Here's how the part is built. I have some questions about the finished solid (model axes, mm). A direction names the side the tool comes from. Coordinates: 2 decimals unless noted, no trailing zeros. Loops run counter-clockwise (first coordinate to the right, second up) from the corner with the lowest first, then second, coordinate; pieces in that order, holes last. Notation, with made-up numbers: M 57,-38 L 105,-38 A16 ccw 105,-11 Z; hole C 56.5,60 d3. An arc over 180 degrees is marked long. Use one line per item in the form item = value. Start each with the question number.
(1) Will this pin go through, and if not, where does the flat tip stop? P1, Ø3.5, axis at x = 41.25, y = -100.5, coming from the +Z side.
(2) Imagine slicing it at A-A, the plane x = 5. Please give me the cut outline in (y, z).
(3) Imagine slicing it at D-D, the plane y = 14.5. Please give me the cut outline in (x, z), and give its area (3 significant figures).
(4) Please list where these lines run through material, in increasing order: L1, parallel to Y at x = 11, z = 1.7; L2, parallel to X at y = -132, z = 0.8; L3, parallel to X at y = 100, z = 0.6.
(5) Imagine slicing it at C-C, the plane z = 2.55. State how many separate pieces and enclosed holes the cut face has, and give its area (3 significant figures).
(6) On a 3-axis mill with a long thin cutter (end or side, diameter ignored), from which of +Z, -Z, +X, -X, +Y, -Y can I reach the whole of each face in a straight line? I mean faces 1 (the flat face through (-37, 3, 0)), 2 (the cylindrical face through (37.591, 9.888, 1.479)). Say none if no direction works.
(7) Thinking about a two-plate mould opening in Y: for faces 3 (the flat face through (-37, 3, 3)), 4 (the cylindrical face through (-37.362, 9.659, 1.479)), which applies, +Y half, -Y half, draft (parallel to the pull), parting line (faces both ways), or undercut?
(8) Imagine slicing it at B-B, the plane y = -57. Please give me the cut outline in (x, z).
Autodesk Inventor part; units mm, degrees
ref_plane "YZ Plane" through (0, 0, 0) normal (1, 0, 0) x (0, 1, 0)
ref_plane "XZ Plane" through (0, 0, 0) normal (0, 1, 0) x (-1, 0, 0)
ref_plane "XY Plane" through (0, 0, 0) normal (0, 0, 1) x (1, 0, 0)
sketch "スケッチ1" plane through (0, 0, 0) normal (0, 0, 1) x (1, 0, 0)
  line L0 (-55, -215) -> (55, -215)
  line L1 (55, -215) -> (55, 215)
  line L2 (55, 215) -> (-55, 215)
  line L3 (-55, 215) -> (-55, -215)
  line L4 (-55, -215) -> (55, 215) construction
  line L5 (55, -215) -> (-55, 215) construction
  line L6 (-55, 185) -> (-50, 185) construction
  line L7 (-50, 185) -> (-25, 210) construction
  line L8 (-25, 210) -> (-25, 215) construction
  line L9 (-46, 95.75) -> (46, 95.75) construction
  line L10 (46, 95.75) -> (46, 187.75) construction
  line L11 (46, 187.75) -> (-46, 187.75) construction
  line L12 (-46, 187.75) -> (-46, 95.75) construction
  line L13 (-46, 95.75) -> (46, 187.75) construction
  line L14 (46, 95.75) -> (-46, 187.75) construction
  line L15 (-46, 1.25) -> (46, 1.25) construction
  line L16 (46, 1.25) -> (46, 93.25) construction
  line L17 (46, 93.25) -> (-46, 93.25) construction
  line L18 (-46, 93.25) -> (-46, 1.25) construction
  line L19 (-46, 1.25) -> (46, 93.25) construction
  line L20 (46, 1.25) -> (-46, 93.25) construction
  line L21 (0, 0) -> (0, 141.75) construction
  circle A0 centre (0, 141.75) radius 53 construction
  line L22 (-44.7, 97.05) -> (44.7, 97.05) construction
  line L23 (44.7, 97.05) -> (44.7, 186.45) construction
  line L24 (44.7, 186.45) -> (-44.7, 186.45) construction
  line L25 (-44.7, 186.45) -> (-44.7, 97.05) construction
  line L26 (-44.7, 97.05) -> (44.7, 186.45) construction
  line L27 (44.7, 97.05) -> (-44.7, 186.45) construction
  arc A1 (-28.4765, 186.45) -> (-44.7, 170.2265) centre (0, 141.75) ccw
  arc A2 (-44.7, 113.2735) -> (-28.4765, 97.05) centre (0, 141.75) ccw
  arc A3 (28.4765, 97.05) -> (44.7, 113.2735) centre (0, 141.75) ccw
  arc A4 (44.7, 170.2265) -> (28.4765, 186.45) centre (0, 141.75) ccw
  line L28 (-28.4765, 186.45) -> (28.4765, 186.45)
  line L29 (-44.7, 170.2265) -> (-44.7, 113.2735)
  line L30 (-28.4765, 97.05) -> (28.4765, 97.05)
  line L31 (44.7, 113.2735) -> (44.7, 170.2265)
  line L32 (-41.25, 100.5) -> (41.25, 100.5) construction
  line L33 (41.25, 100.5) -> (41.25, 183) construction
  line L34 (41.25, 183) -> (-41.25, 183) construction
  line L35 (-41.25, 183) -> (-41.25, 100.5) construction
  line L36 (-41.25, 100.5) -> (41.25, 183) construction
  line L37 (41.25, 100.5) -> (-41.25, 183) construction
  circle A5 centre (-41.25, 183) radius 2.25
  circle A6 centre (-41.25, 100.5) radius 2.25
  circle A7 centre (41.25, 100.5) radius 2.25
  circle A8 centre (41.25, 183) radius 2.25
  circle A9 centre (-41.25, 88.5) radius 2.25
  arc A10 (-28.4765, 91.95) -> (-44.7, 75.7265) centre (0, 47.25) ccw
  line L38 (-28.4765, 91.95) -> (28.4765, 91.95)
  arc A11 (44.7, 75.7265) -> (28.4765, 91.95) centre (0, 47.25) ccw
  circle A12 centre (41.25, 88.5) radius 2.25
  line L39 (44.7, 18.7735) -> (44.7, 75.7265)
  arc A13 (28.4765, 2.55) -> (44.7, 18.7735) centre (0, 47.25) ccw
  circle A14 centre (41.25, 6) radius 2.25
  line L40 (-28.4765, 2.55) -> (28.4765, 2.55)
  circle A15 centre (-41.25, 6) radius 2.25
  arc A16 (-44.7, 18.7735) -> (-28.4765, 2.55) centre (0, 47.25) ccw
  line L41 (-44.7, 75.7265) -> (-44.7, 18.7735)
  circle A17 centre (-41.25, -6) radius 2.25
  arc A18 (-28.4765, -2.55) -> (-44.7, -18.7735) centre (0, -47.25) ccw
  line L42 (-28.4765, -2.55) -> (28.4765, -2.55)
  arc A19 (44.7, -18.7735) -> (28.4765, -2.55) centre (0, -47.25) ccw
  circle A20 centre (41.25, -6) radius 2.25
  line L43 (44.7, -75.7265) -> (44.7, -18.7735)
  arc A21 (28.4765, -91.95) -> (44.7, -75.7265) centre (0, -47.25) ccw
  circle A22 centre (41.25, -88.5) radius 2.25
  line L44 (-28.4765, -91.95) -> (28.4765, -91.95)
  circle A23 centre (-41.25, -88.5) radius 2.25
  arc A24 (-44.7, -75.7265) -> (-28.4765, -91.95) centre (0, -47.25) ccw
  line L45 (-44.7, -18.7735) -> (-44.7, -75.7265)
  circle A25 centre (-41.25, -100.5) radius 2.25
  arc A26 (-28.4765, -97.05) -> (-44.7, -113.2735) centre (0, -141.75) ccw
  line L46 (-28.4765, -97.05) -> (28.4765, -97.05)
  arc A27 (44.7, -113.2735) -> (28.4765, -97.05) centre (0, -141.75) ccw
  circle A28 centre (41.25, -100.5) radius 2.25
  line L47 (44.7, -170.2265) -> (44.7, -113.2735)
  arc A29 (28.4765, -186.45) -> (44.7, -170.2265) centre (0, -141.75) ccw
  circle A30 centre (41.25, -183) radius 2.25
  line L48 (-28.4765, -186.45) -> (28.4765, -186.45)
  circle A31 centre (-41.25, -183) radius 2.25
  arc A32 (-44.7, -170.2265) -> (-28.4765, -186.45) centre (0, -141.75) ccw
  line L49 (-44.7, -113.2735) -> (-44.7, -170.2265)
  circle A33 centre (-45, 205) radius 2.25
  circle A34 centre (45, 205) radius 2.25
  circle A35 centre (45, -205) radius 2.25
  circle A36 centre (-45, -205) radius 2.25
  circle A37 centre (-45, 0) radius 2.25
  circle A38 centre (45, 0) radius 2.25
  line L50 (-55, 0) -> (55, 0) construction
  point P0 (0, 47.25)
  point P1 (0, 47.25)
  dimension "d12" = 106
  dimension "d0" = 110
  dimension "d1" = 430
  dimension "d2" = 135
  dimension "d3" = 30
  dimension "d4" = 30
  dimension "d5" = 5
  dimension "d6" = 92
  dimension "d7" = 92
  dimension "d8" = 92
  dimension "d9" = 92
  dimension "d10" = 2.5
  dimension "d11" = 1.25
  dimension "d13" = 89.4
  dimension "d14" = 89.4
  dimension "d15" = 82.5
  dimension "d16" = 82.5
  dimension "d17" = 4.5
  dimension "d20" = 94.5
  dimension "d25" = 4.5
  dimension "d26" = 10
  dimension "d27" = 10
  dimension "d28" = 10
  dimension "d29" = 10
  dimension "d30" = 10
  dimension "d31" = 10
  dimension "d32" = 10
  dimension "d33" = 10
  dimension "d34" = 10
  dimension "d35" = 10
extrude "押し出し1" add sketch "スケッチ1" along normal blind 3 contours L3 L2 L1 L0 | A37 | A38
sketch "スケッチ2" plane through (0, 0, 3) normal (0, 0, 1) x (1, 0, 0)
  circle A0 centre (-45, 205) radius 2.25 construction
  circle A1 centre (45, -205) radius 2.25 construction
  circle A2 centre (-45, -205) radius 2.25 construction
  circle A3 centre (-43, 203) radius 2.75 construction
  line L0 (55, 215) -> (-55, 215)
  line L1 (-55, 215) -> (-55, -215)
  line L2 (-43.7153, 206.8472) -> (-41.4298, 205.2577)
  line L3 (-45.2577, 201.4298) -> (-46.8472, 203.7153)
  circle A4 centre (-45, 205) radius 2.25 construction
  arc A5 (-43.7153, 206.8472) -> (-46.8472, 203.7153) centre (-45, 205) ccw
  arc A6 (-45.2577, 201.4298) -> (-41.4298, 205.2577) centre (-43, 203) ccw
  line L4 (55, 215) -> (-55, 215) construction
  line L5 (0, 215) -> (0, -215) construction
  line L6 (-55, -215) -> (55, -215) construction
  line L7 (-55, 0) -> (55, 0) construction
  line L8 (55, -215) -> (55, 215) construction
  circle A7 centre (45, 205) radius 2.25 construction
  circle A8 centre (43, 203) radius 2.75 construction
  line L9 (43.7153, 206.8472) -> (41.4298, 205.2577)
  line L10 (45.2577, 201.4298) -> (46.8472, 203.7153)
  circle A9 centre (45, 205) radius 2.25 construction
  arc A10 (46.8472, 203.7153) -> (43.7153, 206.8472) centre (45, 205) ccw
  arc A11 (41.4298, 205.2577) -> (45.2577, 201.4298) centre (43, 203) ccw
  circle A12 centre (-45, -205) radius 2.25 construction
  circle A13 centre (-43, -203) radius 2.75 construction
  line L11 (-43.7153, -206.8472) -> (-41.4298, -205.2577)
  line L12 (-45.2577, -201.4298) -> (-46.8472, -203.7153)
  circle A14 centre (-45, -205) radius 2.25 construction
  arc A15 (-46.8472, -203.7153) -> (-43.7153, -206.8472) centre (-45, -205) ccw
  arc A16 (-41.4298, -205.2577) -> (-45.2577, -201.4298) centre (-43, -203) ccw
  circle A17 centre (45, -205) radius 2.25 construction
  line L13 (45.2577, -201.4298) -> (46.8472, -203.7153)
  arc A18 (45.2577, -201.4298) -> (41.4298, -205.2577) centre (43, -203) ccw
  circle A19 centre (43, -203) radius 2.75 construction
  line L14 (43.7153, -206.8472) -> (41.4298, -205.2577)
  circle A20 centre (45, -205) radius 2.25 construction
  arc A21 (43.7153, -206.8472) -> (46.8472, -203.7153) centre (45, -205) ccw
  point P0 (0, 0)
  dimension "d38" = 5.5
  dimension "d39" = 12
  dimension "d40" = 12
extrude "押し出し2" cut sketch "スケッチ2" against normal through all
equation "\"d4\" = d3"
equation "\"d11\" = 0.5 * d10"
equation "\"d20\" = d7 + d10"
equation "\"d27\" = d26"
equation "\"d28\" = d26"
equation "\"d29\" = d26"
equation "\"d30\" = d26"
equation "\"d31\" = d26"
equation "\"d32\" = d26"
equation "\"d33\" = d26"
equation "\"d34\" = d26"
equation "\"d35\" = d26"
properties part number "front_panel" material "アルミニウム 6061"
Answer:
q1.P1 = through
q2.outline = M -215,0 L -186.45,0 L -186.45,3 L -215,3 Z; M -97.05,0 L -91.95,0 L -91.95,3 L -97.05,3 Z; M -2.55,0 L 2.55,0 L 2.55,3 L -2.55,3 Z; M 91.95,0 L 97.05,0 L 97.05,3 L 91.95,3 Z; M 186.45,0 L 215,0 L 215,3 L 186.45,3 Z
q3.outline = M -55,0 L -41.67,0 L -41.67,3 L -55,3 Z; M 41.67,0 L 55,0 L 55,3 L 41.67,3 Z
q3.area = 80.0 mm²
q4.L1 = -215 to -186.45, -97.05 to -91.95, -2.55 to 2.55, 91.95 to 97.05, 186.45 to 215
q4.L2 = -55 to -44.7, 44.7 to 55
q4.L3 = -55 to -43.44, -39.06 to -32.65, 32.65 to 39.06, 43.44 to 55
q5.separate_pieces = 1
q5.enclosed_holes = 24
q5.area = 16,700 mm²
q6.face_1 = -Z, +X, -X, +Y, -Y
q6.face_2 = +Z, -Z
q7.face_3 = draft
q7.face_4 = undercut
q8.outline = M -55,0 L -44.7,0 L -44.7,3 L -55,3 Z; M 44.7,0 L 55,0 L 55,3 L 44.7,3 Z
